Autodesk Inventor part; units mm, degrees
ref_plane "YZ Plane" through (0, 0, 0) normal (1, 0, 0) x (0, 1, 0)
ref_plane "XZ Plane" through (0, 0, 0) normal (0, 1, 0) x (-1, 0, 0)
ref_plane "XY Plane" through (0, 0, 0) normal (0, 0, 1) x (1, 0, 0)
sketch "Sketch1" plane through (0, 0, 0) normal (0, 0, 1) x (1, 0, 0)
  circle A0 centre (0, 0) radius 6
  dimension "d0" = 12
extrude "Extrusion1" add sketch "Sketch1" along normal mid plane 52.5
sketch "Sketch2" plane through (0, 0, 26.25) normal (0, 0, 1) x (1, 0, 0)
  circle A0 centre (0, 0) radius 6
  line L0 (-4, 4) -> (4, 4)
  line L1 (4, 4) -> (4, -4)
  line L2 (4, -4) -> (-4, -4)
  line L3 (-4, -4) -> (-4, 4)
  line L4 (-4, 4) -> (4, -4) construction
  line L5 (4, 4) -> (-4, -4) construction
  dimension "d3" = 12
  dimension "d4" = 8
  dimension "d5" = 8
extrude "Extrusion2" add sketch "Sketch2" along normal blind 1.5 and the other way blind 34 contours L0 L1 L2 L3
sketch "Sketch6" plane through (0, 0, -26.25) normal (0, 0, -1) x (-1, 0, 0)
  circle A0 centre (0, -4) radius 1.5
  point P0 (0, 0)
  dimension "d28" = 3
  dimension "d29" = 4
hole "Hole2" at (0, -4, -26.25) direction (0, 0, 1) diameter 3.242 depth 11.8 tip angle 118 counterbore diameter 9 counterbore depth 0
sketch "Sketch7" plane through (0, 0, -26.25) normal (0, 0, -1) x (-1, 0, 0)
  point P0 (0, 0)
pattern_circular "Circular Pattern1" count 2 over 360 about axis through (0, 0, 0) along (0, 0, 1) of "Hole2"
sketch "Sketch8" plane through (0, 0, 27.75) normal (0, 0, 1) x (1, 0, 0)
  circle A0 centre (0, 0) radius 1.2628
hole "Hole3" at (0, 0, 27.75) direction (0, 0, -1) diameter 4.134 depth 14.2 tip angle 118
chamfer "Chamfer1" distance 0.5 angle 45 1 edges at (0, 2.067, 27.75)
properties part number "Joint1_Shaft"
Here's how the part is built. I have some questions about the finished solid (model axes, mm). A direction names the side the tool comes from. Coordinates: 2 decimals unless noted, no trailing zeros. Order: outer loops, then holes, each group sorted by start corner. A loop starts at its lowest first (then second) coordinate and runs counter-clockwise, first axis right, second up.
1) Imagine slicing it at A-A on z = -19. List the corners of the cut face in (x, y) for me, and give its area (3 significant figures).
2) Imagine slicing it at D-D on x = 5. List the corners of the cut face in (y, z) for me, and give its area (3 significant figures).
3) I need wall thicknesses on line 1 (Y direction, x = 0, z = 22.25); line 2 (Y direction, x = 0.5, z = -19); line 3 (X direction, y = -4, z = -20). Which ranges of each line are inside material? Lowest first, please.
4) Which directions (+Z, -Z, +X, -X, +Y, -Y) give clear straight access to the entire face, cutting with the end or side of a thin tool? Please do faces 1 (the face through (-4, 0, 27)), 2 (the face through (0, -4, 27)), 3 (the face through (0.07, 5.62, -20.27)).
5) Imagine slicing it at C-C on x = -4.5. List the corners of the cut face in (y, z) for me, and give its area (3 significant figures).
6) We'd pull the mould along X, two halves only. Please class faces 4 (the face through (0, 4, 27)), 5 (the face through (1.26, 1.64, 20.3)), 6 (the face through (-0.012, 4.281, -13.645)), 7 (the face through (4, 0, 27)): +X half, -X half, draft (parallel to the pull), parting line (faces both ways), or undercut.
7) Imagine slicing it at B-B on z = 1.5. List the corners of the cut face in (x, y) for me.
8) Will these pins go through, and if not, where does the flat tip stop? pin 1 (0.8 mm diameter, centred on y = 0, z = 27, fed in from +X); pin 2 (3 mm diameter, centred on y = -4.5, z = 1, fed in from +X); pin 3 (1 mm diameter, centred on y = -1.5, z = -5, fed in from +X).
Response values:
1. outline: circle Ø12 at (0, 0); hole circle Ø3.24 at (0, -4); hole circle Ø3.24 at (0, 4)
1. area: 96.6 mm2
2. outline: (-3.32, -26.25) - (3.32, -26.25) - (3.32, 26.25) - (-3.32, 26.25) - close
2. area: 348 mm2
3. line 1: y = -6 to -2.07, 2.07 to 6
3. line 2: y = -5.98 to -5.54, -2.46 to 2.46, 5.54 to 5.98
3. line 3: x = -4.47 to -1.62, 1.62 to 4.47
4. face 1: +Z, -X, +Y, -Y
4. face 2: +Z, +X, -X, -Y
4. face 3: -Z
5. outline: (-3.97, -26.25) - (3.97, -26.25) - (3.97, 26.25) - (-3.97, 26.25) - close
5. area: 417 mm2
6. face 4: draft
6. face 5: undercut
6. face 6: undercut
6. face 7: +X half
7. outline: circle Ø12 at (0, 0)
8. pin 1: stops at x = 4
8. pin 2: stops at x = 5.2
8. pin 3: stops at x = 5.92
